Can you work these out from the model? Positions are in its coordinate system, mm. Face numbers are marked on the shaded views. Give positions to 0.01 mm unless a question says otherwise; leave off trailing zeros. Loops run counter-clockwise (first coordinate to the right, second up) from the corner with the lowest first, then second, coordinate; pieces in that order, holes last. Notation, with made-up numbers: M 31,-28 L 40,-28 A17 cw 40,-22 Z; hole C 59,-17 d7. An arc over 180 degrees is marked long. Put each result on its own line as item: value. Start each with the question number.
1) Imagine slicing it at B-B (z = -45.9). Write out the boundary of the cut face in (x, y).
2) Imagine slicing it at C-C (z = 40.75). Write out the boundary of the cut face in (x, y), then the cut area to 3 significant figures.
3) Imagine slicing it at A-A (y = 0). Write out the boundary of the cut face in (x, z).
4) If we mould it in two halves opening along X, with no side actions, what happens to the marked faces 1 and 2? For each: +X half, -X half, draft (parallel to the pull), parting line (faces both ways), or undercut.
5) Please list where these lines run through material, in increasing order: line 1 along Z through (x, y) = (1.9, 0); line 2 along Z through (x, y) = (4, -16.22). Write a range as from..to.
6) Imagine slicing it at D-D (y = 16.22). Write out the boundary of the cut face in (x, z).
from build123d import *

# Parameters (mm, degrees)
SKETCH1_W           = 80
SKETCH1_H           = 125
SKETCH1_R           = 5
SKETCH1_R_2         = 1.5
SKETCH1_R_3         = 2.866822522
BOSS_EXTRUDE1_DEPTH = 5


with BuildPart() as part:
    # Sketch1 → Boss-Extrude1 (new body)
    with BuildSketch(Plane.YZ):
        Rectangle(SKETCH1_W, SKETCH1_H)
        with Locations((0, 40.75)):
            Circle(SKETCH1_R, mode=Mode.SUBTRACT)
        with Locations((-16.22, 40.75)):
            Circle(SKETCH1_R_2, mode=Mode.SUBTRACT)
        with Locations((16.22, 40.75)):
            Circle(SKETCH1_R_2, mode=Mode.SUBTRACT)
        with Locations((-25, -45.9)):
            Circle(SKETCH1_R_3, mode=Mode.SUBTRACT)
        with Locations((25, -45.9)):
            Circle(SKETCH1_R_3, mode=Mode.SUBTRACT)
    extrude(amount=BOSS_EXTRUDE1_DEPTH)


solid = part.part
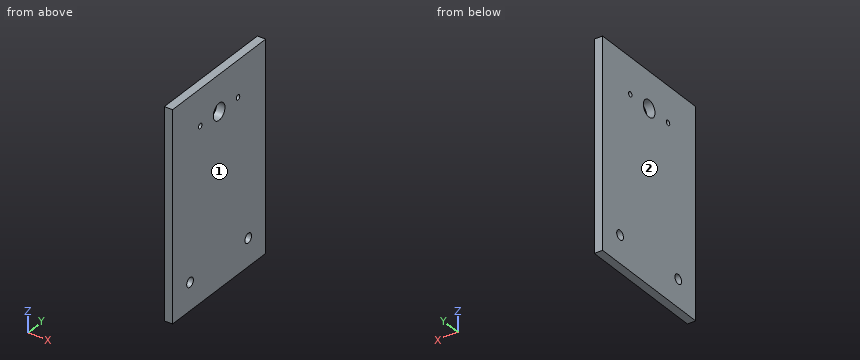
Recorded:
1. outline: M 0,-40 L 5,-40 L 5,-27.87 L 0,-27.87 Z; M 0,-22.13 L 5,-22.13 L 5,22.13 L 0,22.13 Z; M 0,27.87 L 5,27.87 L 5,40 L 0,40 Z
2. outline: M 0,-40 L 5,-40 L 5,-17.72 L 0,-17.72 Z; M 0,-14.72 L 5,-14.72 L 5,-5 L 0,-5 Z; M 0,5 L 5,5 L 5,14.72 L 0,14.72 Z; M 0,17.72 L 5,17.72 L 5,40 L 0,40 Z
2. area: 320 mm²
3. outline: M 0,-62.5 L 5,-62.5 L 5,35.75 L 0,35.75 Z; M 0,45.75 L 5,45.75 L 5,62.5 L 0,62.5 Z
4. face 1: +X half
4. face 2: -X half
5. line 1: -62.5..35.75, 45.75..62.5
5. line 2: -62.5..39.25, 42.25..62.5
6. outline: M 0,-62.5 L 5,-62.5 L 5,39.25 L 0,39.25 Z; M 0,42.25 L 5,42.25 L 5,62.5 L 0,62.5 Z
